Verification items for the finished model (mm, model axes). Round coordinates to 2 decimals unless told otherwise and drop trailing zeros. Order: outer loops, then holes, each group sorted by start corner. A loop starts at its lowest first (then second) coordinate and runs counter-clockwise, first axis right, second up. Notation, with made-up numbers: M 37.5,7 L 90.5,7 A23 cw 90.5,17 Z; hole C -17.75,60 d9. An arc over 180 degrees is marked long. One line per item, written item: value. Start each with the question number.
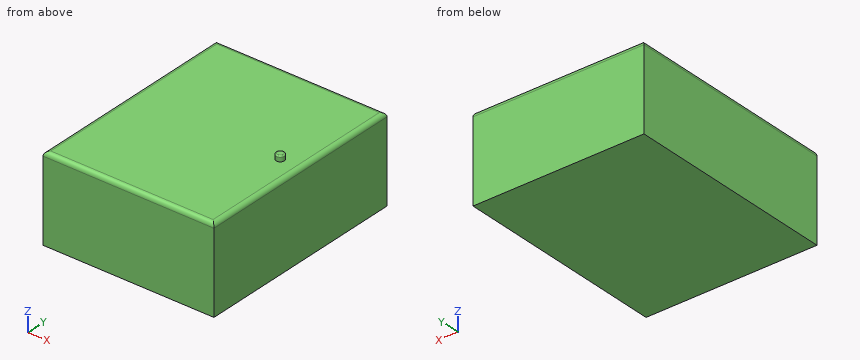
from build123d import *

# Parameters (mm, degrees)
CROQUIS1_W              = 400
CROQUIS1_H              = 500
SALIENTE_EXTRUIR1_DEPTH = 200
REDONDEO1_R             = 10
CROQUIS2_R              = 10
SALIENTE_EXTRUIR2_DEPTH = 12.7
REDONDEO2_R             = 3


with BuildPart() as part:
    # Croquis1 → Saliente-Extruir1 (new body)
    with BuildSketch(Plane.XY):
        with Locations((200, 250)):
            Rectangle(CROQUIS1_W, CROQUIS1_H)
    extrude(amount=SALIENTE_EXTRUIR1_DEPTH)

    # Redondeo1
    redondeo1_edges = [part.edges().sort_by_distance(p)[0] for p in [
        (400, 250, 200),
        (200, 500, 200),
        (0, 250, 200),
        (200, 0, 200),
    ]]
    fillet(redondeo1_edges, radius=REDONDEO1_R)

    # Croquis2 → Saliente-Extruir2 (add)
    with BuildSketch(Plane.XY.offset(200)):
        with Locations(Location((351.956210027, 250.916140829, 0), (0, 0, 180))):
            Circle(CROQUIS2_R)
    extrude(amount=SALIENTE_EXTRUIR2_DEPTH)

    # Redondeo2
    redondeo2_edges = [part.edges().sort_by_distance(p)[0] for p in [
        (361.956210027, 250.916140829, 212.7),
    ]]
    fillet(redondeo2_edges, radius=REDONDEO2_R)


solid = part.part
1. Section check B-B (y = 315). Record the cut outline in (x, z), and give its area (3 significant figures).
2. Section check A-A (x = 104.5). Record the cut outline in (y, z), and give its area (4 significant figures).
3. Depth check by flat-ended pin: pin 1 (3 mm diameter, centred on x = 279.5, y = 284, fed in from +Z). Enter the tip coordinate at first touch or a pass-through.
4. Scan lines: line 1 along Z through (x, y) = (260, 206); line 2 along X through (y, z) = (221.5, 195.5); line 3 along X through (y, z) = (207, 195). Record each from-to range of solid material in increasing order.
Geometry check:
1. outline: M 0,0 L 400,0 L 400,190 A10 ccw 390,200 L 10,200 A10 ccw 0,190 Z
1. area: 80,000 mm²
2. outline: M 0,0 L 500,0 L 500,190 A10 ccw 490,200 L 10,200 A10 ccw 0,190 Z
2. area: 100,000 mm²
3. pin 1: stops at z = 200
4. line 1: z = 0 to 200
4. line 2: x = 1.65 to 398.35
4. line 3: x = 1.34 to 398.66
